Here's the drawing with two shaded views (mm, measured from the low corner). I have some questions. Coordinates: 2 decimals unless noted, no trailing zeros. Write each loop counter-clockwise with the first axis right and the second up, starting at its lowest first coordinate (ties: lowest second). Pieces come first, ordered by that corner, then holes.
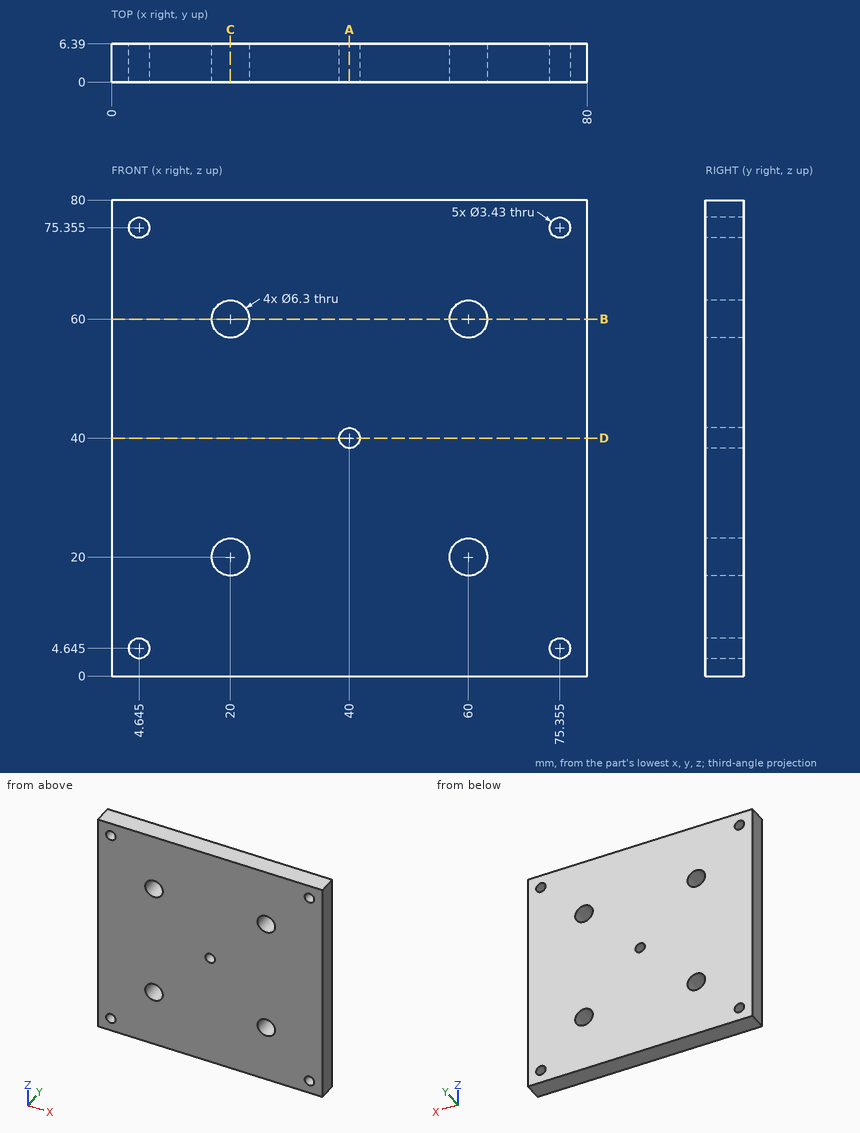
Item 1: I want a section at A-A, the plane x = 40. List the corners of the cut face in (y, z) for me (1 decimal).
Item 2: If I drill on line 1 along Z through (x, y) = (60, 3); line 2 along X through (y, z) = (5.5, 18) (1 decimal); line 3 along X through (y, z) = (5.25, 4) (1 decimal), over which ranges is the centre line in solid material (lowest first)?
Item 3: I want a section at B-B, the plane z = 60. List the corners of the cut face in (x, y) for me, then the cut area to 3 significant figures.
Item 4: Will this pin go through, and if not, where does the flat tip stop? pin 1 Ø5 at (x, z) = (60, 20) entering from +Y.
Item 5: I want a section at C-C, the plane x = 20. List the corners of the cut face in (y, z) for me.
Item 6: I want a section at D-D, the plane z = 40. List the corners of the cut face in (x, y) for me (1 decimal), then the cut area to 3 significant figures.
Taken from the geometry:
1. outline: (0, 0) - (6.4, 0) - (6.4, 38.3) - (0, 38.3) - close; (0, 41.7) - (6.4, 41.7) - (6.4, 80) - (0, 80) - close
2. line 1: z = 0 to 16.85, 23.15 to 56.85, 63.15 to 80
2. line 2: x = 0 to 17.6, 22.4 to 57.6, 62.4 to 80
2. line 3: x = 0 to 3.1, 6.2 to 73.8, 76.9 to 80
3. outline: (0, 0) - (16.85, 0) - (16.85, 6.39) - (0, 6.39) - close; (23.15, 0) - (56.85, 0) - (56.85, 6.39) - (23.15, 6.39) - close; (63.15, 0) - (80, 0) - (80, 6.39) - (63.15, 6.39) - close
3. area: 431 mm2
4. pin 1: passes through
5. outline: (0, 0) - (6.39, 0) - (6.39, 16.85) - (0, 16.85) - close; (0, 23.15) - (6.39, 23.15) - (6.39, 56.85) - (0, 56.85) - close; (0, 63.15) - (6.39, 63.15) - (6.39, 80) - (0, 80) - close
6. outline: (0, 0) - (38.3, 0) - (38.3, 6.4) - (0, 6.4) - close; (41.7, 0) - (80, 0) - (80, 6.4) - (41.7, 6.4) - close
6. area: 489 mm2
